Autodesk Inventor part; units mm, degrees
ref_plane "YZ Plane" through (0, 0, 0) normal (1, 0, 0) x (0, 1, 0)
ref_plane "XZ Plane" through (0, 0, 0) normal (0, 1, 0) x (-1, 0, 0)
ref_plane "XY Plane" through (0, 0, 0) normal (0, 0, 1) x (1, 0, 0)
sketch "草圖1" plane through (0, 0, 0) normal (1, 0, 0) x (0, 1, 0)
  line L0 (-2.97, -1.859) -> (2.97, -1.859)
  line L1 (2.97, -1.859) -> (2.97, 1.859)
  line L2 (2.97, 1.859) -> (-2.97, 1.859)
  line L3 (-2.97, 1.859) -> (-2.97, -1.859)
  line L4 (-2.97, -1.859) -> (2.97, 1.859) construction
  line L5 (2.97, -1.859) -> (-2.97, 1.859) construction
  circle A0 centre (0, 1.859) radius 2.97
  circle A1 centre (0, -1.859) radius 2.97
  line L6 (-2.2651, -3.78) -> (-2.2651, 3.78) construction
  point P0 (0, 0)
  point P1 (-2.97, 1.859)
  dimension "d0" = 7.56
  dimension "d1" = 5.94
extrude "擠出1" add sketch "草圖1" along normal blind 20
sketch "草圖2" plane through (0, 0, 0) normal (0, 0, 1) x (1, 0, 0)
  line L0 (0, 2.4) -> (9, 2.4)
  line L1 (9, 2.4) -> (9, -2.4)
  line L2 (9, -2.4) -> (0, -2.4)
  line L3 (0, -2.4) -> (0, 2.4)
  line L4 (0, -2.97) -> (0, 2.97)
  circle A0 centre (2.4, 0) radius 2.4
  line L5 (9, 5) -> (20, 5)
  line L6 (20, 5) -> (20, -5)
  line L7 (20, -5) -> (9, -5)
  line L8 (9, -5) -> (9, 5)
  line L9 (0, -2.97) -> (0, 2.97)
  line L10 (0, 2.97) -> (20, 2.97)
  line L11 (20, -2.97) -> (20, 2.97)
  line L12 (0, -2.97) -> (20, -2.97)
  arc A1 (7.6018, 2.4) -> (9, 2.97) centre (7.6018, 4.4) ccw
  arc A2 (9, -2.97) -> (7.6018, -2.4) centre (7.6018, -4.4) ccw
  point P0 (0, 0)
  point P1 (0, 0)
  point P2 (9, 0)
  point P3 (2.4, 2.4)
  point P4 (2.4, -2.4)
  dimension "d4" = 4.8
  dimension "d5" = 9
  dimension "d6" = 2
  dimension "d7" = 2
extrude "擠出2" cut sketch "草圖2" along normal mid plane 20 contours A1 L8 L0 | L0 L1 L2 A0 | L8 L10 L6 L12 L1 | A0 | L8 L5 L6 L10 | L8 A2 L2 | L12 L6 L7 L8 keep common part
sketch "草圖3" plane through (0, 0, 0) normal (0, 0, 1) x (1, 0, 0)
  line L0 (-0.1991, -1.7797) -> (-0.0573, 1.9709)
  arc A0 (-0.1991, -1.7797) -> (-0.0573, 1.9709) centre (2.4, 0) ccw
  point P0 (0, 0)
extrude "擠出3" cut sketch "草圖3" along normal mid plane 0.84
sketch "草圖4" plane through (20, 0, 0) normal (1, 0, 0) x (0, 0, -1)
  line L0 (1.859, 2.97) -> (-1.859, 2.97)
  arc A0 (-1.859, 2.97) -> (-1.859, -2.97) centre (-1.859, 0) ccw
  line L1 (-1.859, -2.97) -> (1.859, -2.97)
  arc A1 (1.859, -2.97) -> (1.859, 2.97) centre (1.859, 0) ccw
  line L2 (1.859, 2.38) -> (-1.859, 2.38)
  arc A2 (-1.859, 2.38) -> (-1.859, -2.38) centre (-1.859, 0) ccw
  line L3 (-1.859, -2.38) -> (1.859, -2.38)
  arc A3 (1.859, -2.38) -> (1.859, 2.38) centre (1.859, 0) ccw
  point P0 (0, 0)
  dimension "d14" = 0.59
extrude "擠出4" add sketch "草圖4" along normal blind 4.88 contours A3 L3 A2 L2
sketch "草圖5" plane through (24.88, 0, 0) normal (1, 0, 0) x (0, 0, -1)
  circle A0 centre (0, 0) radius 1.7
  dimension "d17" = 3.4
sketch "草圖6" plane through (0, 0, 0) normal (0, 0, 1) x (1, 0, 0)
  line L0 (24.88, -1.7) -> (24.88, 1.7)
  line L1 (24.88, 0) -> (29.88, 0)
  arc A0 (39.88, -10) -> (29.88, 0) centre (29.88, -10) ccw
  line L2 (39.88, -10) -> (39.88, -30)
  point P0 (0, 0)
  dimension "d18" = 5
  dimension "d19" = 10
  dimension "d20" = 20
sweep "掃掠1" add profiles "草圖5" path "草圖6" path curves L1 A0 L2
properties part number "基座"
The listing builds one solid part. Answer for the finished solid, in the listing's coordinates (mm). A direction names the side the tool comes from. Coordinates: 2 decimals unless noted, no trailing zeros. Loops run counter-clockwise (first coordinate to the right, second up) from the corner with the lowest first, then second, coordinate; pieces in that order, holes last. Notation, with made-up numbers: (-39, 84.25) -> (2, 84.25) arc R30 cw to (2, 122.25) -> close; hole circle Ø6 at (-24, 35). An arc over 180 degrees is marked (long way). Use one line per item in the form item = value. Start each with the question number.
Item 1: Flat-ended cylindrical pins translate along their axes: pin 1 Ø1.5 at (y, z) = (-15.5, 1.5) entering from +X; pin 2 Ø1.4 at (y, z) = (-1, -1.5) entering from +X; pin 3 Ø1.5 at (x, z) = (34, -0.5) entering from -Y. Find the tip coordinate at first contact, or state that the pin passes through.
Item 2: The part is cut by section B-B on x = 5. Determine the outline of the cut face in (y, z), then the cut area to 3 significant figures.
Item 3: The mould has two halves that part along Z. Classify faces 1 (the face through (27.42, -1.66, 0.37)), 2 (the face through (3, 0, 0.42)), 3 (the face through (5.55, 0.04, -0.01)), 4 (the face through (5, 2.4, 0)): released by +Z, released by -Z, zero draft, split by the parting line, or undercut.
Item 4: Consider L1, parallel to Y at x = 12.5, z = 1; L2, parallel to Y at x = 5.5, z = -2.75; L3, parallel to X at y = -19.5, z = 0.25. Determine where each line is inside the solid, lowest interval first. Write a range as [from, to].
Item 5: The part is cut by section D-D on x = 20.5. Determine the outline of the cut face in (y, z), then the cut area to 3 significant figures.
Item 6: A tool of negligible diameter and unlimited length cuts with its end or side. For faces 5 (the face through (5, -2.4, 0)), 6 (the face through (22.41, -0.05, 4.24)), 7 (the face through (41.566, -20.14, 0.221)), 8 (the face through (22, 2.38, 0)), 9 (the face through (22.41, 0.05, -4.24)), from which of +Z, -Z, +X, -X, +Y, -Y can it reach the whole face along a straight path? Write none if from no direction.
Item 7: The part is cut by section A-A on z = -2.75. Determine the outline of the cut face in (x, y).
Item 8: The part is cut by section C-C on y = -21. Determine the outline of the cut face in (x, z), then the cut area to 3 significant figures.
Answer key:
q1.pin_1 = 41.41
q1.pin_2 = 37.43
q1.pin_3 = -3.23
q2.outline = (-2.4, -3.61) arc R2.97 ccw to (2.4, -3.61) -> (2.4, 3.61) arc R2.97 ccw to (-2.4, 3.61) -> close; hole (-1.78, -0.42) -> (1.78, -0.42) -> (1.78, 0.42) -> (-1.78, 0.42) -> close
q2.area = 39.9 mm2
q3.face_1 = split by the parting line
q3.face_2 = undercut
q3.face_3 = undercut
q3.face_4 = zero draft
q4.L1 = [-2.97, 2.97]
q4.L2 = [-2.4, 2.4]
q4.L3 = [38.2, 41.56]
q5.outline = (-2.38, -1.86) arc R2.38 ccw to (2.38, -1.86) -> (2.38, 1.86) arc R2.38 ccw to (-2.38, 1.86) -> close
q5.area = 35.5 mm2
q6.face_5 = +Z, -Z, -X, -Y
q6.face_6 = +Z, +X
q6.face_7 = -Y
q6.face_8 = +Z, -Z, +X, +Y
q6.face_9 = -Z, +X
q7.outline = (2.4, -2.4) -> (7.6, -2.4) arc R2 cw to (8.84, -2.83) -> (20, -2.83) -> (20, -2.21) -> (24.88, -2.21) -> (24.88, 2.21) -> (20, 2.21) -> (20, 2.83) -> (8.84, 2.83) arc R2 cw to (7.6, 2.4) -> (2.4, 2.4) arc R2.4 ccw to start
q8.outline = circle Ø3.4 at (39.88, 0)
q8.area = 9.08 mm2
